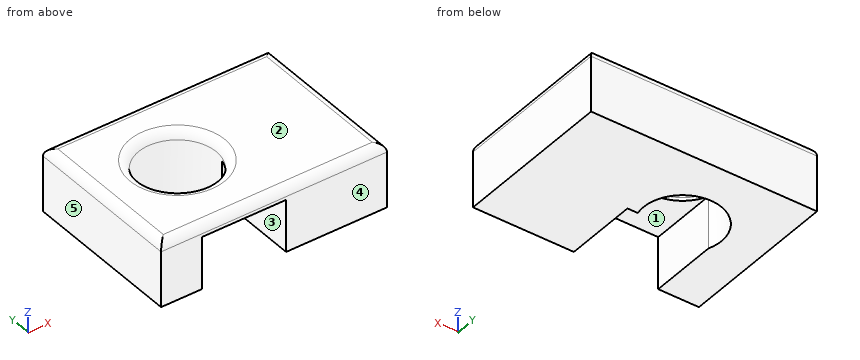
```python
from build123d import *

# Parameters (mm, degrees)
F1_W     = 134.2979371548
F1_H     = 95.1243713498
F1_R     = 23.0942820745
F2_DEPTH = 38.1
F3_W     = 50.118137151
F3_H     = 31.0858320445
F4_DEPTH = 43.18
F5_R     = 5.08


with BuildPart() as f2:
    # F1 (on face) → F2 (new body)
    with BuildSketch(Plane.XY):
        with Locations((21.4310362935, -1.2426972389)):
            Rectangle(F1_W, F1_H)
        Circle(F1_R, mode=Mode.SUBTRACT)
    extrude(amount=F2_DEPTH)

    # F3 (on face) → F4 (cut)
    with BuildSketch(Plane.XZ.offset(48.8048829138)):
        with Locations((3.5529956222, 15.5429160222)):
            Rectangle(F3_W, F3_H)
    extrude(amount=-F4_DEPTH, mode=Mode.SUBTRACT)

    # F5
    f5_edges = [f2.edges().sort_by_distance(p)[0] for p in [
        (21.431036, 46.319488, 38.1),
        (-45.717932, -1.242697, 38.1),
        (21.431036, -48.804883, 38.1),
        (88.580005, -1.242697, 38.1),
        (-23.094282, 0, 38.1),
    ]]
    fillet(f5_edges, radius=F5_R)


solid = f2.part
```
Geometry: final body of the model. Coordinates: model frame, mm. Face numbers are marked on the shaded views. A direction names the side the tool comes from. Round coordinates to 2 decimals unless told otherwise and drop trailing zeros. Order: outer loops, then holes, each group sorted by start corner. A loop starts at its lowest first (then second) coordinate and runs counter-clockwise, first axis right, second up. Notation, with made-up numbers: (79.5, 6) -> (105.5, 6) arc R20 ccw to (105.5, 42) -> close; hole circle Ø6 at (49, -6). An arc over 180 degrees is marked (long way). Use CSV: the item, a comma, the result in double quotes. Start each with the question number.
1) Material intervals for line 1 along X through (y, z) = (0, 20); line 2 along X through (y, z) = (-34, 19); line 3 along Y through (x, z) = (0, 21.5), sorted ascending. Write a range as from..to.
2) Section A-A (y = 0). Return the cut outline in (x, z), and give its area (3 significant figures).
3) First-contact query: pin 1 Ø1.5 at (x, z) = (1, 18.5) entering from -Y; pin 2 Ø1.9 at (x, z) = (24, 11) entering from -Y. Flat tips, straight axial feed; report the tip coordinate or a pass-through.
4) Section C-C (z = 18). Return the cut outline in (x, y), and give its area (3 significant figures).
5) Section D-D (y = -37). Return the cut outline in (x, z), and give its area (3 significant figures).
6) Draft query along X for the marked faces 3, 4 and 5. Return one class per face: +X half, -X half, draft (parallel to the pull), parting line (faces both ways), or undercut.
7) Section B-B (x = 0). Return the cut outline in (y, z), and give its area (3 significant figures).
8) Set-up query: the marked faces 1 and 2. Return all of +Z, -Z, +X, -X, +Y, -Y with unobstructed straight access to the full face (end or side cutting, diameter ignored); none if empty.
Returned:
1,line 1,"x = -45.72..-23.09, 23.09..88.58"
1,line 2,"x = -45.72..-21.51, 28.61..88.58"
1,line 3,"y = 23.09..46.32"
2,outline,"(-45.72, 0) -> (-23.09, 0) -> (-23.09, 33.02) arc R5.08 ccw to (-28.17, 38.1) -> (-40.64, 38.1) arc R5.08 ccw to (-45.72, 33.02) -> close; (23.09, 0) -> (88.58, 0) -> (88.58, 33.02) arc R5.08 ccw to (83.5, 38.1) -> (28.17, 38.1) arc R5.08 ccw to (23.09, 33.02) -> close"
2,area,"3,330 mm²"
3,pin 1,"stops at y = 23.03"
3,pin 2,"stops at y = -5.62"
4,outline,"(-45.72, -48.8) -> (-21.51, -48.8) -> (-21.51, -8.42) arc R23.09 cw (long way) to (22.4, -5.62) -> (28.61, -5.62) -> (28.61, -48.8) -> (88.58, -48.8) -> (88.58, 46.32) -> (-45.72, 46.32) -> close"
4,area,"9,510 mm²"
5,outline,"(-45.72, 0) -> (-21.51, 0) -> (-21.51, 31.09) -> (28.61, 31.09) -> (28.61, 0) -> (88.58, 0) -> (88.58, 33.02) arc R5.08 ccw to (83.5, 38.1) -> (-40.64, 38.1) arc R5.08 ccw to (-45.72, 33.02) -> close"
5,area,"3,550 mm²"
6,face 3,"undercut"
6,face 4,"draft"
6,face 5,"-X half"
7,outline,"(-48.8, 31.09) -> (-23.09, 31.09) -> (-23.09, 33.02) arc R5.08 ccw to (-28.17, 38.1) -> (-43.72, 38.1) arc R5.08 ccw to (-48.8, 33.02) -> close; (23.09, 0) -> (46.32, 0) -> (46.32, 33.02) arc R5.08 ccw to (41.24, 38.1) -> (28.17, 38.1) arc R5.08 ccw to (23.09, 33.02) -> close"
7,area,"1,040 mm²"
8,face 1,"-Z, -Y"
8,face 2,"+Z, +X, -X, +Y, -Y"
